Work out the finished part from the listing and answer in its coordinate system (mm). A direction names the side the tool comes from. Coordinates: 2 decimals unless noted, no trailing zeros. Loops run counter-clockwise (first coordinate to the right, second up) from the corner with the lowest first, then second, coordinate; pieces in that order, holes last. Notation, with made-up numbers: M 46.5,-25.75 L 98.5,-25.75 A27 ccw 98.5,10.25 Z; hole C 57,-39.5 d9. An arc over 180 degrees is marked long. Write each question's results on one line, items separated by ' | '.
```python
from build123d import *

# Parameters (mm, degrees)
SKETCH1_W               = 8
SKETCH1_H               = 8
BOSS_EXTRUDE1_DEPTH     = 3
CUT_EXTRUDE1_DEPTH      = 12.704699911
CUT_EXTRUDE1_DEPTH_BACK = 12.704699911
CUT_EXTRUDE2_DEPTH      = 11
SKETCH4_R               = 1.8
CUT_EXTRUDE3_DEPTH      = 0.8
SKETCH5_W               = 8
SKETCH5_H               = 1
BOSS_EXTRUDE2_DEPTH     = 2
FILLET1_R               = 4
CUT_EXTRUDE4_DEPTH      = 0.4
CUT_EXTRUDE5_DEPTH      = 0.4


with BuildPart() as part:
    # Sketch1 → Boss-Extrude1 (new body)
    with BuildSketch(Plane(origin=(0, 0, 0), x_dir=(1, 0, 0), z_dir=(0, 1, 0))):
        with Locations((4, 4)):
            Rectangle(SKETCH1_W, SKETCH1_H)
    extrude(amount=BOSS_EXTRUDE1_DEPTH)

    # Sketch2 → Cut-Extrude1 (cut, two sides: drawn at the far end of the back side and taken through both)
    with BuildSketch(Plane.XY.offset(-CUT_EXTRUDE1_DEPTH_BACK)):
        Polygon((0, 0), (0.6, 3), (0, 3), align=None)
        Polygon((8, 0), (7.4, 3), (8, 3), align=None)
    extrude(amount=CUT_EXTRUDE1_DEPTH + CUT_EXTRUDE1_DEPTH_BACK, mode=Mode.SUBTRACT)

    # Sketch3 → Cut-Extrude2 (cut)
    with BuildSketch(Plane(origin=(0, 0, 0), x_dir=(0, 0, -1), z_dir=(1, 0, 0))):
        Polygon((0, 0), (0.6, 3), (0, 3), align=None)
        Polygon((8, 3), (7.4, 3), (8, 0), align=None)
    extrude(amount=CUT_EXTRUDE2_DEPTH, mode=Mode.SUBTRACT)

    # Sketch4 → Cut-Extrude3 (cut)
    with BuildSketch(Plane.XZ):
        with Locations(Location((4, -3.75, 0), (0, 0, 270))):
            Circle(SKETCH4_R)
    extrude(amount=-CUT_EXTRUDE3_DEPTH, mode=Mode.SUBTRACT)

    # Sketch5 → Boss-Extrude2 (add)
    with BuildSketch(Plane.XZ):
        with Locations((4, -7.5)):
            Rectangle(SKETCH5_W, SKETCH5_H)
    extrude(amount=BOSS_EXTRUDE2_DEPTH)

    # Fillet1
    # the kernel refuses this fillet: 4 mm, written as the material it takes off along each edge
    with BuildSketch(Plane(origin=(8, -2, -16.660254038), x_dir=(0, 1, 0), z_dir=(0, 0, 1)), Plane(origin=(0, -2, 1.660254038), x_dir=(0, 1, 0), z_dir=(0, 0, -1))) as fillet1_piece_1:
        with BuildLine():
            CenterArc((4, 3.464101615), FILLET1_R, 180, 60)
            Line((0, 3.464101615), (-0.08, 3.464101615))
            Line((-0.08, 3.464101615), (-0.08, 0))
            Line((-0.08, 0), (0, -0.08))
            ThreePointArc((0, -0.08), (1, -0.08), (1.96, -0.069282032))
            Line((1.96, -0.069282032), (2, 0))
        make_face()
    extrude(amount=18.320508076, mode=Mode.SUBTRACT)

    # Sketch6 → Cut-Extrude4 (cut)
    with BuildSketch(Plane(origin=(0, 3, 0), x_dir=(1, 0, 0), z_dir=(0, 1, 0))):
        Polygon((2.459405501, 2.064543337), (2.459405501, 6.064543337), (3.22863627, 6.064543337), (3.22863627, 4.474799747), (4.869661911, 4.474799747), (4.869661911, 6.064543337), (5.63889268, 6.064543337), (5.63889268, 2.064543337), (4.869661911, 2.064543337), (4.869661911, 3.80813308), (3.22863627, 3.80813308), (3.22863627, 2.064543337), align=None)
    extrude(amount=-CUT_EXTRUDE4_DEPTH, mode=Mode.SUBTRACT)

    # Sketch7 → Cut-Extrude5 (cut)
    with BuildSketch(Plane(origin=(0, 3, 0), x_dir=(1, 0, 0), z_dir=(0, 1, 0))):
        Polygon((6.693034442, 1.488274187), (6.626528032, 1.86447611), (6.626528032, 2.206222905), (7.011143417, 2.206222905), (7.011143417, 1.86447611), (6.953451109, 1.488274187), align=None)
    extrude(amount=-CUT_EXTRUDE5_DEPTH, mode=Mode.SUBTRACT)


solid = part.part
```
1) Find section B-B, the plane x = 4. Give the vertices of the cut face in (y, z), and give its area (3 significant figures).
Check result:
outline: M -2,-8 L 0,-8 L 3,-7.4 L 3,-4.47 L 2.6,-4.47 L 2.6,-3.81 L 3,-3.81 L 3,-0.6 L 0,0 L 0,-1.95 L 0.8,-1.95 L 0.8,-5.55 L 0,-5.55 L 0,-7 L -2,-7 Z | area: 21.1 mm^2
2) Find section A-A, the plane z = -7.25. Give the vertices of the cut face in (x, y), and give its area (3 significant figures).
Check result:
outline: M 0,0 A4 ccw 3.46,-2 L 4.54,-2 A4 ccw 8,0 L 7.4,3 L 0.6,3 Z | area: 34.2 mm^2
3) Which of the six approach directions +Z, -Z, +X, -X, +Y, -Y give full straight-line access (tool end or side, diameter ignored) to faces 5 (the face through (4, 0.8, -4)), 6 (the face through (6.51, -1.48, -7.51)), 7 (the face through (4, -1, -7))?
Check result:
face 5: -Y | face 6: +Z, -Z, +X, -Y | face 7: +Z, +X, -X, -Y
4) Find section C-C, the plane y = 2.2. Give the vertices of the cut face in (x, z).
Check result:
outline: M 0.44,-7.56 L 7.56,-7.56 L 7.56,-0.44 L 0.44,-0.44 Z
5) Find section D-D, the plane z = -0.75. Give the vertices of the cut face in (x, y).
Check result:
outline: M 0,0 L 8,0 L 7.4,3 L 0.6,3 Z
6) Given pin 1 Ø3 at (x, y) = (5.5, 2) entering from -Z; pin 2 Ø3 at (y, z) = (-0.5, -2.5) entering from +X; pin 3 Ø2 at (y, z) = (2, -5) entering from -X, each flat-ended and moving along its own axis, determine where each tip first touches the part or whether it passes through.
Check result:
pin 1: z = -7.9 | pin 2: x = 8 | pin 3: x = 0.2
7) Straight lines are drawn through the part: probe 1 along Y at (x, z) = (6.25, -1); probe 2 along Y at (x, z) = (5.5, -3.5); probe 3 along X at (y, z) = (0.65, -3.75). For each, find the intervals that lie inside material, in ascending order. Write a range as [from, to].
Check result:
probe 1: [0, 3] | probe 2: [0.8, 2.6] | probe 3: [0.13, 2.2], [5.8, 7.87]
8) For a pull along X with two mould halves and no side action, classify faces 1 (the face through (0.3, 1.5, -4.1)), 2 (the face through (4, 2.6, -4)), 3 (the face through (3.9, 1.5, -0.3)), 4 (the face through (7.7, 1.5, -4.1)) as released by +X, released by -X, zero draft, split by the parting line, or undercut.
Check result:
face 1: released by -X | face 2: undercut | face 3: zero draft | face 4: released by +X
